Check sheet for the modelled part. Datum: model origin and axes. Units: mm. Coordinates: 2 decimals unless noted, no trailing zeros. Loops run counter-clockwise (first coordinate to the right, second up) from the corner with the lowest first, then second, coordinate; pieces in that order, holes last.
Autodesk Inventor part; units mm, degrees
ref_plane "YZ Plane" through (0, 0, 0) normal (1, 0, 0) x (0, 1, 0)
ref_plane "XZ Plane" through (0, 0, 0) normal (0, 1, 0) x (-1, 0, 0)
ref_plane "XY Plane" through (0, 0, 0) normal (0, 0, 1) x (1, 0, 0)
sketch "Sketch1" plane through (0, 0, 0) normal (0, 0, 1) x (1, 0, 0)
  circle A0 centre (0, 0) radius 245
  circle A1 centre (0, 0) radius 285
  circle A2 centre (0, 0) radius 265 construction
  line L0 (0, 285) -> (0, 245) construction
  point P0 (0, 265)
  dimension "d9" = 530
  dimension "d11" = 40
extrude "Plate1" add sketch "Sketch1" along normal blind 3
sketch "Sketch2" plane through (0, 0, 3) normal (0, 0, 1) x (1, 0, 0)
  circle A0 centre (0, 0) radius 245 construction
  circle A1 centre (0, 0) radius 285 construction
  circle A2 centre (0, 0) radius 285
  circle A3 centre (0, 0) radius 245
  line L0 (0, 0) -> (0, -285) construction
  line L1 (0, 0) -> (-55.6007, -279.5238) construction
  line L2 (-47.7971, -240.2924) -> (-55.6007, -279.5238) construction
  circle A4 centre (-51.6989, -259.9081) radius 6
  dimension "d20" = 11.25
  dimension "d21" = 12
extrude "Extrusion1" cut sketch "Sketch2" against normal through all contours A4
sketch "Sketch3" plane through (0, 0, 3) normal (0, 0, 1) x (1, 0, 0)
  circle A0 centre (0, 0) radius 245
  line L0 (-245, 0) -> (-250, 0) construction
  line L1 (-250, 5) -> (-250, -5)
  line L2 (-250, 5) -> (-244.949, 5)
  line L3 (-250, -5) -> (-244.949, -5)
  line L4 (245, 0) -> (250, 0) construction
  line L5 (250, 5) -> (250, -5)
  line L6 (250, 5) -> (244.949, 5)
  line L7 (250, -5) -> (244.949, -5)
  dimension "d23" = 5
  dimension "d24" = 10
extrude "Extrusion2" [suppressed]
pattern_circular "Circular Pattern2" count 16 over 360 about axis through (0, 0, 0) along (0, 0, 1) of "Extrusion1"
equation "\"d9\" = Шпил_пласт_КОРМА_диам_центров"
equation "\"d11\" = Шпил_пласт_КОРМА_ширина"
equation "\"d21\" = Шпил_пласт_КОРМА_диам_шпильки"
equation "\"d2\" = Thickness"
equation "\"BendRadius\" = Thickness"
equation "\"BendReliefWidth\" = Thickness"
equation "\"BendReliefDepth\" = 0.5 * Thickness"
equation "\"CornerReliefSize\" = 4 * Thickness"
equation "\"MinimumRemnant\" = 2 * Thickness"
equation "\"TransitionRadius\" = BendRadius"
equation "\"JacobiRadiusSize\" = BendRadius"
equation "\"GapSize\" = Thickness"
properties part number "ДМФ 041 кольцо под шпильки КОРМА v2.0"
1) Depth check by flat-ended pin: pin 1 (1 mm diameter, centred on y = -50, z = 2.5, fed in from +X). Enter the tip coordinate at first touch or a pass-through.
Answer sheet:
pin 1: stops at x = 280.67
2) Scan lines: line 1 (X direction, y = -6.5, z = 1.15); line 2 (X direction, y = -219, z = 2.65); line 3 (X direction, y = -258, z = 0.7). Record each from-to range of solid material in increasing order.
Answer sheet:
line 1: x = -284.93 to -244.91, 244.91 to 284.93
line 2: x = -182.38 to -153.07, -141.38 to -109.84, 109.84 to 141.38, 153.07 to 182.38
line 3: x = -121.08 to -57.39, -46.01 to 46.01, 57.39 to 121.08
3) Section check A-A on y = 0. Enter the section's corners in (x, z), plus the area to 3 significant figures.
Answer sheet:
outline: (-285, 0) - (-245, 0) - (-245, 3) - (-285, 3) - close; (245, 0) - (285, 0) - (285, 3) - (245, 3) - close
area: 240 mm2
4) Mould release check, pull along X, two halves, no side actions. Record for faces 1 (the flat face through (125, 212, 3)), 2 (the cylindrical face through (-53.111, 239.174, 1.479)), 3 (the cylindrical face through (-210.057, -192.617, 1.479)): +X half, -X half, draft (parallel to the pull), parting line (faces both ways), or undercut.
Answer sheet:
face 1: draft
face 2: undercut
face 3: parting line
